```python
from build123d import *

# Parameters (mm, degrees)
CHAMFER1_SIZE  = 0.47037037
CHAMFER1_SIZE2 = 0.81470538


with BuildPart() as part:
    # Sketch1 → Revolve1 (revolve)
    with BuildSketch(Plane.XY):
        Polygon((0, 0), (-9.5377, 0), (-9.5377, 4.7625), (-8.001, 4.7625), (-8.001, 7.14375), (-9.5377, 7.14375), (-9.5377, 9.525), (0, 9.525), align=None)
    revolve(axis=Axis((0, 0, 0), (0, 1, 0)))

    # Chamfer1
    chamfer1_edges = [part.edges().sort_by_distance(p)[0] for p in [
        (9.5377, 9.525, 0),
    ]]
    chamfer1_side = [part.faces().sort_by_distance(p)[0] for p in [
        (0, 9.525, 0),
    ]]
    chamfer(chamfer1_edges, length=CHAMFER1_SIZE, length2=CHAMFER1_SIZE2, reference=chamfer1_side[0])


solid = part.part
```
Work out the finished part from the listing and answer in its coordinate system (mm). A direction names the side the tool comes from. Round coordinates to 2 decimals unless told otherwise and drop trailing zeros. Order: outer loops, then holes, each group sorted by start corner. A loop starts at its lowest first (then second) coordinate and runs counter-clockwise, first axis right, second up.
Q1. A cutting plane is placed at A-A, the plane x = 0. Determine the outline of the cut face in (y, z) (1 decimal), then the cut area to 3 significant figures.
Solution:
outline: (0, -9.5) - (4.8, -9.5) - (4.8, -8) - (7.1, -8) - (7.1, -9.5) - (8.7, -9.5) - (9.5, -9.1) - (9.5, 9.1) - (8.7, 9.5) - (7.1, 9.5) - (7.1, 8) - (4.8, 8) - (4.8, 9.5) - (0, 9.5) - close
area: 174 mm2
Q2. A cutting plane is placed at C-C, the plane y = 8.25. Determine the outline of the cut face in (x, z).
Solution:
outline: circle Ø19.08 at (0, 0)
Q3. Given pin 1 Ø3 at (x, y) = (7, 4.5) entering from -Z; pin 2 Ø2 at (y, z) = (3.5, -5.5) entering from +X; pin 3 Ø3 at (y, z) = (2.5, 5) entering from -X, each flat-ended and moving along its own axis, determine where each tip first touches the part or whether it passes through.
Solution:
pin 1: stops at z = -7.79
pin 2: stops at x = 8.41
pin 3: stops at x = -8.87
Q4. A cutting plane is placed at B-B, the plane z = 0. Determine the outline of the cut face in (x, y) (1 decimal).
Solution:
outline: (-9.5, 0) - (9.5, 0) - (9.5, 4.8) - (8, 4.8) - (8, 7.1) - (9.5, 7.1) - (9.5, 8.7) - (9.1, 9.5) - (-9.1, 9.5) - (-9.5, 8.7) - (-9.5, 7.1) - (-8, 7.1) - (-8, 4.8) - (-9.5, 4.8) - close
Q5. A cutting plane is placed at D-D, the plane y = 6. Determine the outline of the cut face in (x, z).
Solution:
outline: circle Ø16 at (0, 0)
Q6. Find the intervals of material crossed by line 1 along Y through (x, z) = (3, 7.5) (1 decimal); line 2 along Z through (x, y) = (0.25, 8), in increasing order.
Solution:
line 1: y = 0 to 4.8, 7.1 to 9.5
line 2: z = -9.53 to 9.53
Q7. The mould has two halves that part along Y. Classify faces 1 (the cylindrical face through (2.07, 2.41, -9.31)), 2 (the flat face through (-2, 7.144, 8)), 3 (the flat face through (0, 9.525, 0)), 4 (the flat face through (0, 0, 0)): pulls with the +Y half, pulls with the -Y half, needs draft (parallel to the pull), parting line crosses it, or undercut.
Solution:
face 1: needs draft
face 2: undercut
face 3: pulls with the +Y half
face 4: pulls with the -Y half
Q8. A tool of negligible diameter and unlimited length cuts with its end or side. For faces 5 (the flat face through (2, 4.762, 8)), 6 (the cylindrical face through (2.07, 7.94, -9.31)), from which of +Z, -Z, +X, -X, +Y, -Y can it reach the whole face along a straight path? Write none if from no direction.
Solution:
face 5: none
face 6: +Y, -Y
